Autodesk Inventor part; units mm, degrees
ref_plane "Arbeitsebene1" through (0, 0, 180) normal (0, 0, 1) x (1, 0, 0)
ref_plane "YZ Plane" through (0, 0, 0) normal (1, 0, 0) x (0, 1, 0)
ref_plane "XZ Plane" through (0, 0, 0) normal (0, 1, 0) x (-1, 0, 0)
sketch "Skizze1" plane through (0, 0, 0) normal (0, 0, 1) x (1, 0, 0)
  line L0 (0, 0) -> (10, 0)
  line L1 (10, 0) -> (10, 10)
  line L2 (10, 10) -> (0, 10)
  line L3 (0, 10) -> (0, 0)
extrude "Extrusion1" add sketch "Skizze1" along normal blind 180
sketch "Skizze2" plane through (0, 0, 0) normal (0, 0, 1) x (1, 0, 0)
  line L0 (0, 0) -> (4, 0)
  line L1 (4, 0) -> (4, 4)
  line L2 (4, 4) -> (0, 4)
  line L3 (0, 4) -> (0, 0)
extrude "Extrusion2" cut sketch "Skizze2" along normal blind 180
sketch "Skizze3" plane through (0, 0, 0) normal (0, 0, 1) x (1, 0, 0)
  line L0 (-3, 6) -> (3, 6)
  line L1 (3, 6) -> (3, 10)
  line L2 (3, 10) -> (-3, 10)
  line L3 (-3, 10) -> (-3, 6)
extrude "Extrusion3" cut sketch "Skizze3" along normal blind 180
sketch "Skizze4" plane through (0, 0, 0) normal (0, 0, 1) x (1, 0, 0)
  line L0 (-3, -10) -> (3, -10)
  line L1 (3, -10) -> (3, -6)
  line L2 (3, -6) -> (-3, -6)
  line L3 (-3, -6) -> (-3, -10)
extrude "Extrusion4" cut sketch "Skizze4" along normal blind 180
sketch "Skizze5" plane through (0, 0, 0) normal (0, 0, 1) x (1, 0, 0)
  line L0 (-10, -3) -> (-6, -3)
  line L1 (-6, -3) -> (-6, 3)
  line L2 (-6, 3) -> (-10, 3)
  line L3 (-10, 3) -> (-10, -3)
extrude "Extrusion5" cut sketch "Skizze5" along normal blind 180
sketch "Skizze6" plane through (0, 0, 0) normal (0, 0, 1) x (1, 0, 0)
  line L0 (6, -3) -> (10, -3)
  line L1 (10, -3) -> (10, 3)
  line L2 (10, 3) -> (6, 3)
  line L3 (6, 3) -> (6, -3)
extrude "Extrusion6" cut sketch "Skizze6" along normal blind 180
ref_plane "Arbeitsebene1" through (0, 0, 180) normal (0, 0, 1) x (1, 0, 0)
sketch "Skizze7" plane through (0, 0, 0) normal (0, 0, 1) x (1, 0, 0)
  circle A0 centre (0, 0) radius 2.5
extrude "Extrusion7" cut sketch "Skizze7" along normal blind 10
sketch "Skizze8" plane through (0, 0, 180) normal (0, 0, 1) x (1, 0, 0)
  circle A0 centre (0, 0) radius 2.5
extrude "Extrusion8" cut sketch "Skizze8" along normal blind 10
properties part number "Aluprofil_20x20_L180"
Model file for the job. Use its own axes, mm. A direction names the side the tool comes from. Give positions to 0.01 mm unless a question says otherwise; leave off trailing zeros. Order: outer loops, then holes, each group sorted by start corner. A loop starts at its lowest first (then second) coordinate and runs counter-clockwise, first axis right, second up. Notation, with made-up numbers: (68.5, 80.5) - (123.5, 80.5) arc R23 ccw to (123.5, 109.5) - close; hole circle Ø11 at (43.25, -24.75). An arc over 180 degrees is marked (long way). Return JSON: item names as keys, results as strings.
1) Cut at B-B, the plane x = 8.5. Give the cut face in (y, z).
Geometry says:
{"outline": "(3, 0) - (10, 0) - (10, 180) - (3, 180) - close"}
2) Cut at A-A, the plane z = 78.5. Give the cut face in (x, y), plus the area to 3 significant figures.
Geometry says:
{"outline": "(0, 4) - (4, 4) - (4, 0) - (6, 0) - (6, 3) - (10, 3) - (10, 10) - (3, 10) - (3, 6) - (0, 6) - close", "area": "60.0 mm²"}
3) 3-axis set-ups, long thin cutter, end or side, ignore diameter. For faces 1 (the flat face through (1, 6, 89)), 2 (the flat face through (8, 3, 89)), 3 (the flat face through (4, 2, 89)), 4 (the flat face through (6, 6, 180)): which of +Z, -Z, +X, -X, +Y, -Y reach the whole face in a straight line?
Geometry says:
{"face 1": "+Z, -Z, -X, +Y", "face 2": "+Z, -Z, +X, -Y", "face 3": "+Z, -Z, -X, -Y", "face 4": "+Z, +X, -X, +Y, -Y"}
4) Probe line 1 (Y direction, x = 6.5, z = 117); line 2 (Y direction, x = 1.5, z = 124). List the from-to ranges inside material, lowest first. Write a range as from..to.
Geometry says:
{"line 1": "3..10", "line 2": "4..6"}
5) Flat gauge pins, fed straight in: P1, Ø4, axis at x = 5.5, y = 4.5, coming from the -Z side; P2, Ø3, axis at x = 8, z = 50, coming from the -Y side; P3, Ø1.2, axis at x = 2.5, z = 51, coming from the -Y side; P4, Ø0.9, axis at x = 2, z = 100.5, coming from the +Y side. Where does each tip first touch, or does it go through?
Geometry says:
{"P1": "z = 0", "P2": "y = 3", "P3": "y = 4", "P4": "y = 6"}
6) Pull direction Y, two halves, no side cores. Call faces 5 (the flat face through (6, 6, 0)), 6 (the flat face through (2, 4, 89)), 7 (the flat face through (7, 10, 89)): pulls with the +Y half, pulls with the -Y half, needs draft (parallel to the pull), parting line crosses it, or undercut.
Geometry says:
{"face 5": "needs draft", "face 6": "pulls with the -Y half", "face 7": "pulls with the +Y half"}
